Verification items for the finished model (mm, model axes). A direction names the side the tool comes from. Round coordinates to 2 decimals unless told otherwise and drop trailing zeros. Order: outer loops, then holes, each group sorted by start corner. A loop starts at its lowest first (then second) coordinate and runs counter-clockwise, first axis right, second up. Notation, with made-up numbers: (64.25, 17.25) -> (108.25, 17.25) arc R19 ccw to (108.25, 36.25) -> close; hole circle Ø6 at (8.25, -1). An arc over 180 degrees is marked (long way). Return JSON: item names as keys, results as strings. Group by question number.
1) Section check B-B on z = 0. Enter the section's corners in (x, y), plus the area to 3 significant figures.
2) Draft check along X on faces 1 (the flat face through (0.616, 2.014, 1.088)), 2 (the flat face through (-1.5, 3, 0)), 3 (the cylindrical face through (0.596, 1.334, 2.685)). Enter one of: pulls with the +X half, pulls with the -X half, needs draft (parallel to the pull), parting line crosses it, or undercut.
3) Section check A-A on y = 2.25. Enter the section's corners in (x, z), plus the area to 3 significant figures.
4) Scan lines: L1, parallel to Y at x = -0.2, z = 1.8; L2, parallel to Y at x = -1.2, z = -0.4; L3, parallel to Z at x = 0.9, y = 2.5. Record each from-to range of solid material in increasing order.
5) Tool access check on faces 4 (the flat face through (0, -10, 0)), 5 (the flat face through (-2, 0, 0)), 6 (the flat face through (1.25, 2, 0)). Record the directions out of +Z, -Z, +X, -X, +Y, -Y that give a thin tool (end or side, any length) a straight path to the whole face; none if there is none.
6) Depth check by flat-ended pin: pin 1 (0.8 mm diameter, centred on x = 0.5, z = 0, fed in from +Y). Enter the tip coordinate at first touch or a pass-through.
7) Section check C-C on y = -2.5. Enter the section's corners in (x, z).
Autodesk Inventor part; units mm, degrees
ref_plane "YZ Plane" through (0, 0, 0) normal (1, 0, 0) x (0, 1, 0)
ref_plane "XZ Plane" through (0, 0, 0) normal (0, 1, 0) x (-1, 0, 0)
ref_plane "XY Plane" through (0, 0, 0) normal (0, 0, 1) x (1, 0, 0)
sketch "スケッチ1" plane through (0, 0, 0) normal (0, 1, 0) x (-1, 0, 0)
  circle A0 centre (0, 0) radius 2.75
  dimension "d0" = 5.5
extrude "押し出し1" add sketch "スケッチ1" along normal blind 3
sketch "スケッチ2" plane through (0, 0, 0) normal (0, -1, 0) x (1, 0, 0)
  circle A0 centre (0, 0) radius 1.5
  dimension "d3" = 3
extrude "押し出し2" add sketch "スケッチ2" along normal blind 10
fillet "フィレット1" radius 0.5 1 edges at (2.75, 3, 0)
fillet "フィレット1" radius 0.2 1 edges at (2.75, 0, 0)
sketch "スケッチ3" plane through (0, 3, 0) normal (0, 1, 0) x (1, 0, 0)
  line L0 (0, 1.4434) -> (-1.25, 0.7217)
  line L1 (-1.25, 0.7217) -> (-1.25, -0.7217)
  line L2 (-1.25, -0.7217) -> (0, -1.4434)
  line L3 (0, -1.4434) -> (1.25, -0.7217)
  line L4 (1.25, -0.7217) -> (1.25, 0.7217)
  line L5 (1.25, 0.7217) -> (0, 1.4434)
  line L6 (0, 1.4434) -> (0, -1.4434) construction
  circle A0 centre (0, 0) radius 1.4434 construction
  dimension "d12" = 2.5
extrude "押し出し3" cut sketch "スケッチ3" against normal blind 2
thread "ねじ1"
properties part number "M3-CapScrew"
Check result:
{
 "1": {"outline": "(-2.75, 0.2) arc R0.2 ccw to (-2.55, 0) -> (-1.5, 0) -> (-1.5, -10) -> (1.5, -10) -> (1.5, 0) -> (2.55, 0) arc R0.2 ccw to (2.75, 0.2) -> (2.75, 2.5) arc R0.5 ccw to (2.25, 3) -> (1.25, 3) -> (1.25, 1) -> (-1.25, 1) -> (-1.25, 3) -> (-2.25, 3) arc R0.5 ccw to (-2.75, 2.5) -> close", "area": "41.4 mm^2"},
 "2": {"face 1": "undercut", "face 2": "needs draft", "face 3": "parting line crosses it"},
 "3": {"outline": "circle Ø5.5 at (0, 0); hole (-1.25, -0.72) -> (0, -1.44) -> (1.25, -0.72) -> (1.25, 0.72) -> (0, 1.44) -> (-1.25, 0.72) -> close", "area": "18.3 mm^2"},
 "4": {"L1": "0 to 3", "L2": "-10 to 1", "L3": "-2.6 to -0.92, 0.92 to 2.6"},
 "5": {"face 4": "+Z, -Z, +X, -X, -Y", "face 5": "-Y", "face 6": "+Y"},
 "6": {"pin 1": "y = 1"},
 "7": {"outline": "circle Ø3 at (0, 0)"}
}
